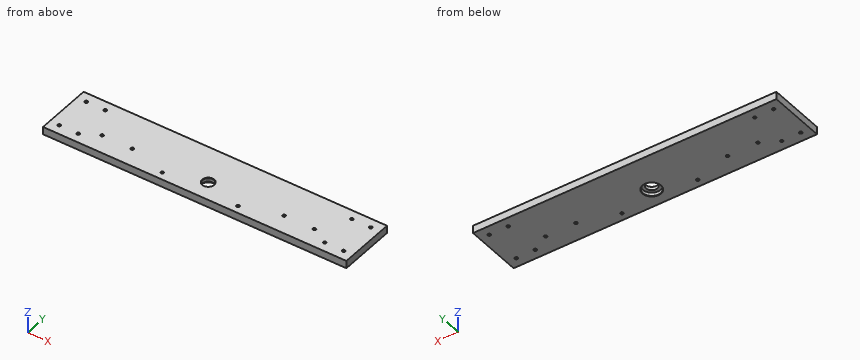
Solid Edge part; units mm, degrees
sketch "Sketch1" plane through (0, 0, 0) normal (0, 0, 1) x (1, 0, 0)
  line L0 (400, 150) -> (-400, 150)
  line L1 (-400, 150) -> (-400, 0)
  line L2 (-400, 0) -> (400, 0)
  line L3 (400, 0) -> (400, 150)
extrude "Protrusion1" add sketch "Sketch1" along normal blind 20
hole "Hole1" at (-280, 50, 20) direction (0, 0, -1) diameter 6 end through all start chamfer 1 start chamfer angle 45 end chamfer 1 end chamfer angle 45
hole "Hole2" at (-200, 50, 20) direction (0, 0, -1) diameter 6 end through all start chamfer 1 start chamfer angle 45 end chamfer 1 end chamfer angle 45
hole "Hole3" at (280, 50, 20) direction (0, 0, -1) diameter 6 end through all start chamfer 1 start chamfer angle 45 end chamfer 1 end chamfer angle 45
hole "Hole4" at (200, 50, 20) direction (0, 0, -1) diameter 6 end through all start chamfer 1 start chamfer angle 45 end chamfer 1 end chamfer angle 45
hole "Hole5" at (-375, 125, 20) direction (0, 0, -1) diameter 6 end through all start chamfer 1 start chamfer angle 45 end chamfer 1 end chamfer angle 45
hole "Hole6" at (-325, 125, 20) direction (0, 0, -1) diameter 6 end through all start chamfer 1 start chamfer angle 45 end chamfer 1 end chamfer angle 45
hole "Hole7" at (-325, 25, 20) direction (0, 0, -1) diameter 6 end through all start chamfer 1 start chamfer angle 45 end chamfer 1 end chamfer angle 45
hole "Hole8" at (-375, 25, 20) direction (0, 0, -1) diameter 6 end through all start chamfer 1 start chamfer angle 45 end chamfer 1 end chamfer angle 45
hole "Hole9" at (325, 125, 20) direction (0, 0, -1) diameter 6 end through all start chamfer 1 start chamfer angle 45 end chamfer 1 end chamfer angle 45
hole "Hole10" at (375, 125, 20) direction (0, 0, -1) diameter 6 end through all start chamfer 1 start chamfer angle 45 end chamfer 1 end chamfer angle 45
hole "Hole11" at (375, 25, 20) direction (0, 0, -1) diameter 6 end through all start chamfer 1 start chamfer angle 45 end chamfer 1 end chamfer angle 45
hole "Hole12" at (325, 25, 20) direction (0, 0, -1) diameter 6 end through all start chamfer 1 start chamfer angle 45 end chamfer 1 end chamfer angle 45
hole "Hole13" at (-100, 20, 20) direction (0, 0, -1) diameter 6 end through all start chamfer 1 start chamfer angle 45 end chamfer 1 end chamfer angle 45
hole "Hole14" at (100, 20, 20) direction (0, 0, -1) diameter 6 end through all start chamfer 1 start chamfer angle 45 end chamfer 1 end chamfer angle 45
hole "Stufenbohrung_Radiallager" at (0, 50, 0) direction (0, 0, 1) diameter 30 end through all counterbore diameter 47 counterbore depth 10 start chamfer 1 start chamfer angle 45 end chamfer 1 end chamfer angle 45
The model under review builds one solid part; all positions refer to its coordinate system, in mm. Round coordinates to 2 decimals unless told otherwise and drop trailing zeros. Write each loop counter-clockwise with the first axis right and the second up, starting at its lowest first coordinate (ties: lowest second). Pieces come first, ordered by that corner, then holes. Notation, with made-up numbers: (-4, 89.25) -> (9, 89.25) arc R13 cw to (9, 94.25) -> close; hole circle Ø11 at (84.25, 5). An arc over 180 degrees is marked (long way). Use CSV: the item, a comma, the result in double quotes.
Q1. To check wall thickness, follow probe 1 along X at (y, z) = (25, 15); probe 2 along Y at (x, z) = (-280, 14.75); probe 3 along X at (y, z) = (50, 15.5). State the ranges of each line that lie inside material, in increasing order. Write a range as [from, to].
Checks:
probe 1,"[-400, -378], [-372, -328], [-322, 322], [328, 372], [378, 400]"
probe 2,"[0, 47], [53, 150]"
probe 3,"[-400, -283], [-277, -203], [-197, -15], [15, 197], [203, 277], [283, 400]"
Q2. For pin 1 Ø7 at (x, y) = (-100, 20) entering from +Z, flat-tipped, find the tip position at first contact; note if it passes through.
Checks:
pin 1,"z = 19.5"
Q3. Consider section A-A (x = 0). Give the boundary of the cut face in (y, z).
Checks:
outline,"(0, 0) -> (25.5, 0) -> (26.5, 1) -> (26.5, 10) -> (35, 10) -> (35, 19) -> (34, 20) -> (0, 20) -> close; (65, 10) -> (73.5, 10) -> (73.5, 1) -> (74.5, 0) -> (150, 0) -> (150, 20) -> (66, 20) -> (65, 19) -> close"
